Input: part model. Units: mm. Frame: model coordinates. A direction names the side the tool comes from. Coordinates: 2 decimals unless noted, no trailing zeros. Order: outer loops, then holes, each group sorted by start corner. A loop starts at its lowest first (then second) coordinate and runs counter-clockwise, first axis right, second up. Notation, with made-up numbers: (5.25, -39) -> (15.25, -39) arc R21 ccw to (15.25, -4) -> close; hole circle Ø4 at (-8.5, -7.5). An arc over 180 degrees is marked (long way). One line per item, written item: value. Start each with the question number.
from build123d import *

# Parameters (mm, degrees)
ESQUISSE1_W             = 4
ESQUISSE1_H             = 4
BOSS_EXTRU_1_DEPTH      = 4
ENL_V_MAT_EXTRU_1_REACH = 14.845
CONG_2_R                = 1.5


with BuildPart() as part:
    # Esquisse1 → Boss.-Extru.1 (new body)
    with BuildSketch(Plane.XY):
        with BuildLine():
            Line((0, 0), (6, 0))
            Line((6, 0), (6, -4))
            Line((6, -4), (7, -4))
            Line((7, -4), (7, -9.166666667))
            ThreePointArc((7, -9.166666667), (6.755922318, -9.755922318), (6.166666667, -10))
            Line((6.166666667, -10), (-0.166666667, -10))
            ThreePointArc((-0.166666667, -10), (-0.755922318, -9.755922318), (-1, -9.166666667))
            Line((-1, -9.166666667), (-1, -4))
            Line((-1, -4), (0, -4))
            Line((0, -4), (0, 0))
        make_face()
        with Locations((3, -6)):
            Rectangle(ESQUISSE1_W, ESQUISSE1_H, mode=Mode.SUBTRACT)
    extrude(amount=BOSS_EXTRU_1_DEPTH)

    # Esquisse2 → Enlèv. mat.-Extru.1 (cut, up to next)
    with BuildSketch(Plane.XY.offset(4), mode=Mode.PRIVATE) as enl_v_mat_extru_1_sk1:
        Polygon((0, 0), (0, -10.686908442), (-3.147637421, -9.875475315), (-3.03761259, -0.798426774), align=None)
    enl_v_mat_extru_1_tool1 = extrude(enl_v_mat_extru_1_sk1.sketch, amount=-ENL_V_MAT_EXTRU_1_REACH, mode=Mode.PRIVATE) & part.part
    add(enl_v_mat_extru_1_tool1.solids().sort_by_distance((-1.504511, -5.371974, 4))[0], mode=Mode.SUBTRACT)

    # Congé2
    cong_2_edges = [part.edges().sort_by_distance(p)[0] for p in [
        (0, -10, 2),
    ]]
    fillet(cong_2_edges, radius=CONG_2_R)


solid = part.part
1) Ray query, line 1 along Y through (x, z) = (3.25, 3.15); line 2 along X through (y, z) = (-7.5, 1.1); line 3 along X through (y, z) = (-2.25, 3.7). Return the intervals inside material, ascending. Write a range as from..to.
2) Access query for faces 1 (the flat face through (3, -8, 2)), 2 (the flat face through (3.5, -3.8, 4)), 3 (the flat face through (6.5, -4, 2)). Directions: +Z, -Z, +X, -X, +Y, -Y. A direction counts if a zero-diameter tool reaches every point of the face in a straight line with its end or side. Return the directions, or none.
3) Section query B-B, the plane x = 3.25. Return the cut outline in (y, z).
4) Section query D-D, the plane y = -1.75. Return the cut outline in (x, z), plus the area to 3 significant figures.
5) Section query A-A, the plane y = -6. Return the cut outline in (x, z).
6) Mould query, pull axis X, two halves, no side actions, for faces 4 (the flat face through (3, -4, 2)), 5 (the flat face through (3, 0, 2)), 6 (the cylindrical face through (6.76, -9.75, 1.97)). Classes: +X half, -X half, draft (parallel to the pull), parting line (faces both ways), or undercut.
7) Section query C-C, the plane z = 1.85. Return the cut outline in (x, y), plus the area to 3 significant figures.
8) Pin query (flat end, axial travel): pin 1 Ø0.5 at (x, z) = (6.5, 2.5) entering from +Y; pin 2 Ø1.2 at (y, z) = (-2.5, 2.5) entering from +X. Return the tip coordinate at first contact, or that it passes through.
Entries:
1. line 1: y = -10..-8, -4..0
1. line 2: x = 0..1, 5..7
1. line 3: x = 0..6
2. face 1: +Z, -Z
2. face 2: +Z, +X, -X, +Y, -Y
2. face 3: +Z, -Z, +X, +Y
3. outline: (-10, 0) -> (-8, 0) -> (-8, 4) -> (-10, 4) -> close; (-4, 0) -> (0, 0) -> (0, 4) -> (-4, 4) -> close
4. outline: (0, 0) -> (6, 0) -> (6, 4) -> (0, 4) -> close
4. area: 24.0 mm2
5. outline: (0, 0) -> (1, 0) -> (1, 4) -> (0, 4) -> close; (5, 0) -> (7, 0) -> (7, 4) -> (5, 4) -> close
6. face 4: undercut
6. face 5: draft
6. face 6: +X half
7. outline: (0, -8.5) arc R1.5 ccw to (1.5, -10) -> (6.17, -10) arc R0.83 ccw to (7, -9.17) -> (7, -4) -> (6, -4) -> (6, 0) -> (0, 0) -> close; hole (1, -8) -> (5, -8) -> (5, -4) -> (1, -4) -> close
7. area: 49.4 mm2
8. pin 1: stops at y = -4
8. pin 2: stops at x = 6
